Check sheet for the modelled part. Datum: model origin and axes. Units: mm. Face numbers are marked on the shaded views. A direction names the side the tool comes from. Round coordinates to 2 decimals unless told otherwise and drop trailing zeros. Loops run counter-clockwise (first coordinate to the right, second up) from the corner with the lowest first, then second, coordinate; pieces in that order, holes last. Notation, with made-up numbers: (-7, 85) -> (48, 85) arc R20 cw to (48, 106) -> close; hole circle Ø1 at (17, 47.5). An arc over 180 degrees is marked (long way). One line per question, with ' | ' between items.
```python
from build123d import *

# Parameters (mm, degrees)
F0_W      = 254
F0_H      = 203.2
F0_R      = 7.14375
F1_DEPTH  = 12.7
F2_W      = 254
F2_H      = 203.2
F2_R      = 7.14375
F3_DEPTH  = 12.7
F4_W      = 254
F4_H      = 12.7
F5_DEPTH  = 50.8
F6_SIZE   = 38.1
F7_W      = 254
F7_H      = 12.7
F8_DEPTH  = 50.8
F9_SIZE   = 38.1
F11_SIZE  = 6.35
F12_W     = 290.5442907095
F12_H     = 101.1743683696
F13_DEPTH = 203.201


with BuildPart() as f1:
    # F0 (on Top) → F1 (new body)
    with BuildSketch(Plane.XY):
        with Locations((-76.2, 0)):
            Rectangle(F0_W, F0_H)
        with Locations((-184.15, -82.55)):
            Circle(F0_R, mode=Mode.SUBTRACT)
        with Locations((-95.25, -82.55)):
            Circle(F0_R, mode=Mode.SUBTRACT)
        with Locations((-184.15, 82.55)):
            Circle(F0_R, mode=Mode.SUBTRACT)
        with Locations((-95.25, 82.55)):
            Circle(F0_R, mode=Mode.SUBTRACT)
    extrude(amount=F1_DEPTH)


with BuildPart() as f3:
    # F2 (on face) → F3 (new body)
    with BuildSketch(Plane(origin=(0, 0, 0), x_dir=(1, 0, 0), z_dir=(0, 0, -1))):
        with Locations((76.2, 0)):
            Rectangle(F2_W, F2_H)
        with Locations((95.25, -82.55)):
            Circle(F2_R, mode=Mode.SUBTRACT)
        with Locations((184.15, -82.55)):
            Circle(F2_R, mode=Mode.SUBTRACT)
        with Locations((95.25, 82.55)):
            Circle(F2_R, mode=Mode.SUBTRACT)
        with Locations((184.15, 82.55)):
            Circle(F2_R, mode=Mode.SUBTRACT)
    extrude(amount=F3_DEPTH)


with BuildPart() as f5:
    # F4 (on face) → F5 (new body)
    with BuildSketch(Plane.XY.offset(12.7)):
        with Locations((-76.2, 0)):
            Rectangle(F4_W, F4_H)
    extrude(amount=F5_DEPTH)

    # F6
    f6_edges = [f5.edges().sort_by_distance(p)[0] for p in [
        (-203.2, 0, 63.5),
        (50.8, 0, 63.5),
    ]]
    chamfer(f6_edges, length=F6_SIZE)


with BuildPart() as f8:
    # F7 (on face) → F8 (new body)
    with BuildSketch(Plane(origin=(0, 0, -12.7), x_dir=(1, 0, 0), z_dir=(0, 0, -1))):
        with Locations((76.2, 0)):
            Rectangle(F7_W, F7_H)
    extrude(amount=F8_DEPTH)

    # F9
    f9_edges = [f8.edges().sort_by_distance(p)[0] for p in [
        (203.2, 0, -63.5),
        (-50.8, 0, -63.5),
    ]]
    chamfer(f9_edges, length=F9_SIZE)


with BuildPart() as f1_1:
    add(f1.part)

    # F10: union F5, F3, F8
    add(f5.part)
    add(f3.part)
    add(f8.part)

    # F11
    f11_edges = [f1_1.edges().sort_by_distance(p)[0] for p in [
        (50.8, 0, 0),
        (-76.2, -6.35, 12.7),
        (-76.2, 6.35, 12.7),
        (-50.8, 0, 0),
        (76.2, 6.35, -12.7),
        (76.2, -6.35, -12.7),
    ]]
    chamfer(f11_edges, length=F11_SIZE)

    # F12 (on face) → F13 (cut, through all)
    with BuildSketch(Plane.XZ.offset(101.6)):
        with Locations((94.4721453547, -63.2871841848)):
            Rectangle(F12_W, F12_H)
    extrude(amount=-F13_DEPTH, mode=Mode.SUBTRACT)


solid = f1_1.part
```
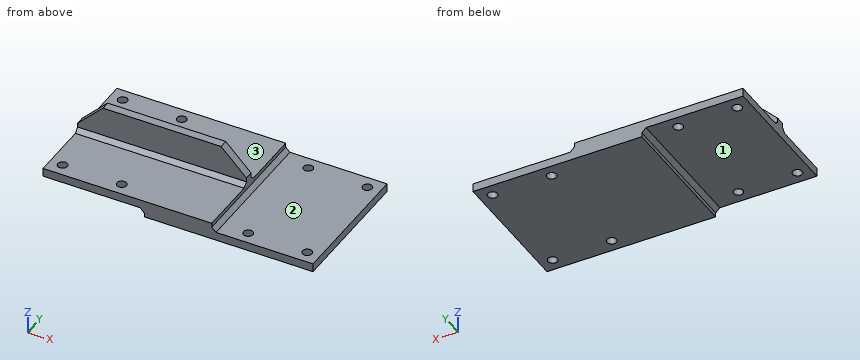
(1) Scan lines: probe 1 along Y at (x, z) = (95, -9); probe 2 along X at (y, z) = (-82, -8); probe 3 along X at (y, z) = (-82, -6). Record each from-to range of solid material in increasing order.
Answer:
probe 1: y = -101.6 to -89.69, -75.41 to 75.41, 89.69 to 101.6 | probe 2: x = -50.8 to 88.13, 102.37 to 177.03, 191.27 to 203.2 | probe 3: x = -51.15 to 88.13, 102.37 to 177.03, 191.27 to 203.2
(2) Set-up check for the marked faces 1, 2 and 3: record each of +Z, -Z, +X, -X, +Y, -Y from which the full face is reachable in a straight line by a thin tool's end or side.
Answer:
face 1: -Z, -X, +Y, -Y | face 2: +Z, +X, +Y, -Y | face 3: +Z, +X, -X, +Y
(3) Go/stop test with flat-tipped pins: pin 1 (23 mm diameter, centred on x = 184.15, y = 82.55, fed in from +Z); pin 2 (18.5 mm diameter, centred on x = -95.25, y = 82.55, fed in from +Z); pin 3 (18.5 mm diameter, centred on x = -184.15, y = 82.55, fed in from -Z); pin 4 (16.5 mm diameter, centred on x = 184.15, y = -82.55, fed in from -Z). Record where each tip stops, or that it passes through.
Answer:
pin 1: stops at z = 0 | pin 2: stops at z = 12.7 | pin 3: stops at z = 0 | pin 4: stops at z = -12.7
(4) Sectioned sample at D-D, the plane z = 35. Record the cut outline in (x, y), and give its area (3 significant figures).
Answer:
outline: (-193.6, -6.35) -> (41.2, -6.35) -> (41.2, 6.35) -> (-193.6, 6.35) -> close | area: 2,980 mm2
(5) Sectioned sample at B-B, the plane y = -82.55. Record the cut outline in (x, z).
Answer:
outline: (-203.2, 0) -> (-191.29, 0) -> (-191.29, 12.7) -> (-203.2, 12.7) -> close; (-177.01, 0) -> (-102.39, 0) -> (-102.39, 12.7) -> (-177.01, 12.7) -> close; (-88.11, 0) -> (-57.15, 0) -> (-50.8, -6.35) -> (-50.8, -12.7) -> (88.11, -12.7) -> (88.11, 0) -> (57.15, 0) -> (50.8, 6.35) -> (50.8, 12.7) -> (-88.11, 12.7) -> close; (102.39, -12.7) -> (177.01, -12.7) -> (177.01, 0) -> (102.39, 0) -> close; (191.29, -12.7) -> (203.2, -12.7) -> (203.2, 0) -> (191.29, 0) -> close
(6) Sectioned sample at C-C, the plane x = 23.5. Record the cut outline in (y, z).
Answer:
outline: (-101.6, -12.7) -> (101.6, -12.7) -> (101.6, 12.7) -> (12.7, 12.7) -> (6.35, 19.05) -> (6.35, 52.7) -> (-6.35, 52.7) -> (-6.35, 19.05) -> (-12.7, 12.7) -> (-101.6, 12.7) -> close
(7) Sectioned sample at A-A, the plane x = 184.15. Record the cut outline in (y, z), and give its area (3 significant figures).
Answer:
outline: (-101.6, -12.7) -> (-89.69, -12.7) -> (-89.69, 0) -> (-101.6, 0) -> close; (-75.41, -12.7) -> (75.41, -12.7) -> (75.41, 0) -> (-75.41, 0) -> close; (89.69, -12.7) -> (101.6, -12.7) -> (101.6, 0) -> (89.69, 0) -> close | area: 2,220 mm2
